Here's how the part is built. I have some questions about the finished solid (model axes, mm). Face numbers are marked on the shaded views. A direction names the side the tool comes from. Coordinates: 2 decimals unless noted, no trailing zeros. Loops run counter-clockwise (first coordinate to the right, second up) from the corner with the lowest first, then second, coordinate; pieces in that order, holes last. Notation, with made-up numbers: M 42,-16.5 L 46,-16.5 A30 ccw 46,6.5 Z; hole C -37,15.25 d1. An arc over 180 degrees is marked long. Use CSV: the item, a comma, the result in double quotes. Start each with the question number.
Q1. Please list where these lines run through material, in increasing order: probe 1 along Y at (x, z) = (-5.4, 24.5); probe 2 along X at (y, z) = (16.75, 9); probe 3 along X at (y, z) = (12.25, -21). Write a range as [from, to].
Q2. For pin 1 Ø3.5 at (y, z) = (12, 22.5) entering from +X; pin 2 Ø2 at (y, z) = (7.5, -25.5) entering from -X; pin 3 Ø6 at (x, y) = (-20, 9) entering from -Z, each with a flat end and sliding along its axis, tell me the tip position at first contact or that it passes through.
Q3. If we section it at B-B (y = 10): Please give me the cut outline in (x, z), and give its area (3 significant figures).
Q4. If we section it at D-D (x = 4): Please give me the cut outline in (y, z), and give its area (3 significant figures).
Q5. Which directions (+Z, -Z, +X, -X, +Y, -Y) give clear straight access to the entire face, cutting with the end or side of a thin tool? Please do the marked faces 1, 2, 3, 4 and 5.
Q6. If we section it at A-A (z = -24.5): Please give me the cut outline in (x, y).
Q7. If we section it at C-C (z = 10): Please give me the cut outline in (x, y).
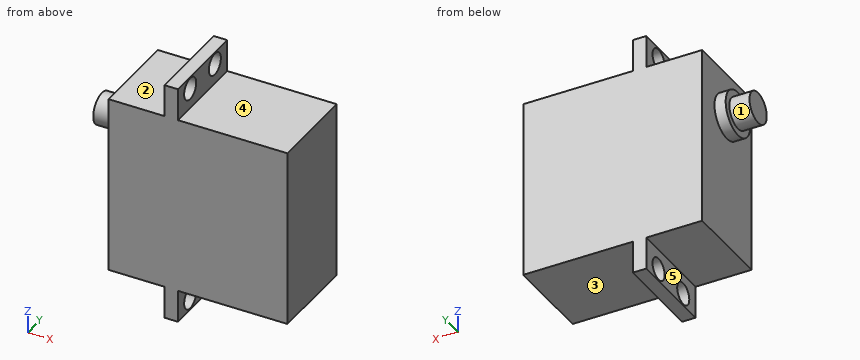
from build123d import *

# Parameters (mm, degrees)
SKETCH_1_W           = 40
SKETCH_1_H           = 40
EXTRUDE_1_DEPTH      = 20
EXTRUDE_2_DEPTH      = 7.25
EXTRUDE_2_DEPTH_BACK = 47.25
SKETCH_4_W           = 3
SKETCH_4_H           = 20
SKETCH_5_R           = 2.45
CUT_EXTRUDE_3_DEPTH  = 7.25
SKETCH_6_R           = 3.5
EXTRUDE_3_DEPTH      = 7
SKETCH_7_R           = 5
EXTRUDE_4_DEPTH      = 2.5


with BuildPart() as part:
    # 草图1 → 凸台-拉伸1 (new body)
    with BuildSketch(Plane(origin=(0, 0, 0), x_dir=(1, 0, 0), z_dir=(0, 1, 0))):
        Rectangle(SKETCH_1_W, SKETCH_1_H)
    extrude(amount=EXTRUDE_1_DEPTH)

    # 草图4 → 凸台-拉伸2 (add, two sides: drawn at the far end of the back side and taken through both)
    with BuildSketch(Plane(origin=(0, 0, -20), x_dir=(-1, 0, 0), z_dir=(0, 0, -1)).offset(-EXTRUDE_2_DEPTH_BACK)):
        with Locations((6, 10)):
            Rectangle(SKETCH_4_W, SKETCH_4_H)
    extrude(amount=EXTRUDE_2_DEPTH + EXTRUDE_2_DEPTH_BACK)

    # 草图5 → 切除-拉伸3 (cut)
    with BuildSketch(Plane.ZY.offset(7.5)):
        with Locations((-24.5, 15)):
            Circle(SKETCH_5_R)
        with Locations((24.5, 15)):
            Circle(SKETCH_5_R)
        with Locations((24.5, 5)):
            Circle(SKETCH_5_R)
        with Locations((-24.5, 5)):
            Circle(SKETCH_5_R)
    extrude(amount=-CUT_EXTRUDE_3_DEPTH, mode=Mode.SUBTRACT)

    # 草图6 → 凸台-拉伸3 (add)
    with BuildSketch(Plane.ZY.offset(20)):
        with Locations(Location((10, 10, 0), (0, 0, 180))):
            Circle(SKETCH_6_R)
    extrude(amount=EXTRUDE_3_DEPTH)

    # 草图7 → 凸台-拉伸4 (add)
    with BuildSketch(Plane.ZY.offset(20)):
        with Locations(Location((10, 10, 0), (0, 0, 180))):
            Circle(SKETCH_7_R)
    extrude(amount=EXTRUDE_4_DEPTH)


solid = part.part
Results below:
1,probe 1,"[0, 2.55], [7.45, 12.55], [17.45, 20]"
1,probe 2,"[-20, 20]"
1,probe 3,"[-7.5, -4.5]"
2,pin 1,"x = -4.5"
2,pin 2,"x = -7.5"
2,pin 3,"z = -20"
3,outline,"M -27,6.5 L -22.5,6.5 L -22.5,5 L -20,5 L -20,-20 L -7.5,-20 L -7.5,-27.25 L -4.5,-27.25 L -4.5,-20 L 20,-20 L 20,20 L -4.5,20 L -4.5,27.25 L -7.5,27.25 L -7.5,20 L -20,20 L -20,15 L -22.5,15 L -22.5,13.5 L -27,13.5 Z"
3,area,"1,700 mm^2"
4,outline,"M 0,-20 L 20,-20 L 20,20 L 0,20 Z"
4,area,"800 mm^2"
5,face 1,"-X"
5,face 2,"+Z, -X, +Y, -Y"
5,face 3,"-Z, +X, +Y, -Y"
5,face 4,"+Z, +X, +Y, -Y"
5,face 5,"-Z, -X, +Y, -Y"
6,outline,"M -7.5,0 L -4.5,0 L -4.5,2.55 L -7.5,2.55 Z; M -7.5,7.45 L -4.5,7.45 L -4.5,12.55 L -7.5,12.55 Z; M -7.5,17.45 L -4.5,17.45 L -4.5,20 L -7.5,20 Z"
7,outline,"M -27,6.5 L -22.5,6.5 L -22.5,5 L -20,5 L -20,0 L 20,0 L 20,20 L -20,20 L -20,15 L -22.5,15 L -22.5,13.5 L -27,13.5 Z"
